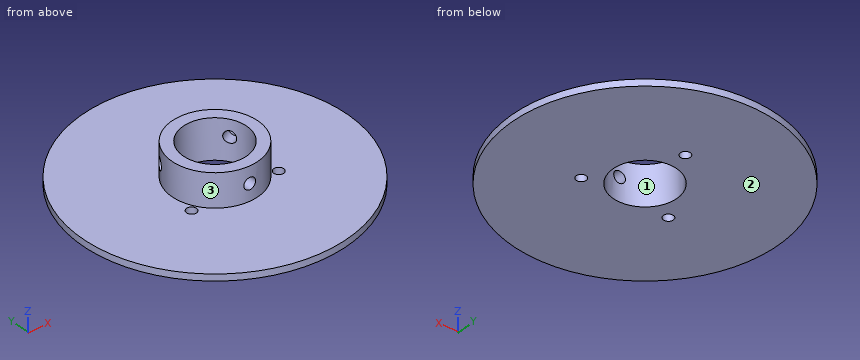
```python
from build123d import *

# Parameters (mm, degrees)
SKETCH1_R           = 40
BOSS_EXTRUDE1_DEPTH = 2
SKETCH2_R           = 13
BOSS_EXTRUDE2_DEPTH = 10
SKETCH3_R           = 9.6
CUT_EXTRUDE1_DEPTH  = 58.827329179
SKETCH4_R           = 1.75
CUT_EXTRUDE2_DEPTH  = 58.827329179
CIRPATTERN1_COUNT   = 3
SKETCH5_R           = 1.5
CUT_EXTRUDE3_DEPTH  = 10
CIRPATTERN2_COUNT   = 3


with BuildPart() as part:
    # Sketch1 → Boss-Extrude1 (new body)
    with BuildSketch(Plane.XY):
        Circle(SKETCH1_R)
    extrude(amount=BOSS_EXTRUDE1_DEPTH)

    # Sketch2 → Boss-Extrude2 (add)
    with BuildSketch(Plane.XY.offset(2)):
        Circle(SKETCH2_R)
    extrude(amount=BOSS_EXTRUDE2_DEPTH)

    # Sketch3 → Cut-Extrude1 (cut, through all)
    with BuildSketch(Plane(origin=(0, 0, 0), x_dir=(-1, 0, 0), z_dir=(0, 0, -1))):
        Circle(SKETCH3_R)
    extrude(amount=-CUT_EXTRUDE1_DEPTH, mode=Mode.SUBTRACT)

    # Sketch4 → Cut-Extrude2 (cut, through all)
    with BuildSketch(Plane(origin=(0, 0, 0), x_dir=(1, 0, 0), z_dir=(0, 1, 0))):
        with Locations(Location((0, -7, 0), (0, 0, 270))):
            Circle(SKETCH4_R)
    cut_extrude2 = extrude(amount=-CUT_EXTRUDE2_DEPTH, mode=Mode.SUBTRACT)

    # CirPattern1: Cut-Extrude2 ×3 about axis
    cirpattern1_axis = Axis((0, 0, 12), (0, 0, -1))
    for i in range(1, CIRPATTERN1_COUNT):
        add(cut_extrude2.rotate(cirpattern1_axis, i * 360 / CIRPATTERN1_COUNT), mode=Mode.SUBTRACT)

    # Sketch5 → Cut-Extrude3 (cut)
    with BuildSketch(Plane(origin=(0, 0, 0), x_dir=(-1, 0, 0), z_dir=(0, 0, -1))):
        with Locations((12.990381057, -7.5)):
            Circle(SKETCH5_R)
    cut_extrude3 = extrude(amount=-CUT_EXTRUDE3_DEPTH, mode=Mode.SUBTRACT)

    # CirPattern2: Cut-Extrude3 ×3 about axis
    cirpattern2_axis = Axis((0, 0, 0), (0, 0, 1))
    for i in range(1, CIRPATTERN2_COUNT):
        add(cut_extrude3.rotate(cirpattern2_axis, i * 360 / CIRPATTERN2_COUNT), mode=Mode.SUBTRACT)


solid = part.part
```
Work out the finished part from the listing and answer in its coordinate system (mm). Face numbers are marked on the shaded views. Give positions to 0.01 mm unless a question says otherwise; leave off trailing zeros. Write each loop counter-clockwise with the first axis right and the second up, starting at its lowest first coordinate (ties: lowest second). Pieces come first, ordered by that corner, then holes. Notation, with made-up numbers: (51.25, 9) - (104.25, 9) arc R23 ccw to (104.25, 23) - close; hole circle Ø4 at (4.25, 43.5). An arc over 180 degrees is marked (long way). Use one line per item in the form item = value.
1. Determine the mould class of the marked faces 1, 2 and 3 for opening direction X: released by +X, released by -X, zero draft, split by the parting line, or undercut.
Filled in:
face_1 = undercut
face_2 = zero draft
face_3 = split by the parting line
2. Consider L1, parallel to Y at x = 0, z = 0.55; L2, parallel to Z at x = 25, y = -14; L3, parallel to X at y = -10.4, z = 7. Determine where each line is inside the solid, lowest interval first.
Filled in:
L1 = -40 to -9.6, 9.6 to 13.5, 16.5 to 40
L2 = 0 to 2
L3 = -7.8 to -1.75, 1.75 to 7.8
3. A cutting plane is placed at B-B (z = 7). Write down the section's boundary in (x, y).
Filled in:
outline = (-12.03, 4.93) arc R13 ccw to (-1.75, -12.88) - (-1.75, -9.44) arc R9.6 cw to (-9.05, 3.2) - close; (-10.28, 7.96) - (-7.3, 6.24) arc R9.6 cw to (7.3, 6.24) - (10.28, 7.96) arc R13 ccw to start; (1.75, -12.88) arc R13 ccw to (12.03, 4.93) - (9.05, 3.2) arc R9.6 cw to (1.75, -9.44) - close
4. A cutting plane is placed at C-C (y = 15). Write down the section's boundary in (x, z).
Filled in:
outline = (-37.08, 0) - (-1.5, 0) - (-1.5, 2) - (-37.08, 2) - close; (1.5, 0) - (37.08, 0) - (37.08, 2) - (1.5, 2) - close
5. A cutting plane is placed at D-D (x = 21). Write down the section's boundary in (y, z), and give its area (3 significant figures).
Filled in:
outline = (-34.04, 0) - (34.04, 0) - (34.04, 2) - (-34.04, 2) - close
area = 136 mm^2
6. Each of these flat-tipped pins is pushed along its axis until it touches: pin 1 Ø2 at (x, z) = (0, 7) entering from -Y; pin 2 Ø3 at (x, z) = (-0.5, 9) entering from +Y; pin 3 Ø2 at (x, z) = (4, 2.5) entering from +Y; pin 4 Ø2.5 at (x, y) = (-12.99, -7.5) entering from -Z. Where does it stop, or does it pass through?
Filled in:
pin_1 = 9.55
pin_2 = 13
pin_3 = 39.88
pin_4 = through
7. A cutting plane is placed at A-A (y = 0). Write down the section's boundary in (x, z).
Filled in:
outline = (-40, 0) - (-9.6, 0) - (-9.6, 12) - (-13, 12) - (-13, 2) - (-40, 2) - close; (9.6, 0) - (40, 0) - (40, 2) - (13, 2) - (13, 12) - (9.6, 12) - close
